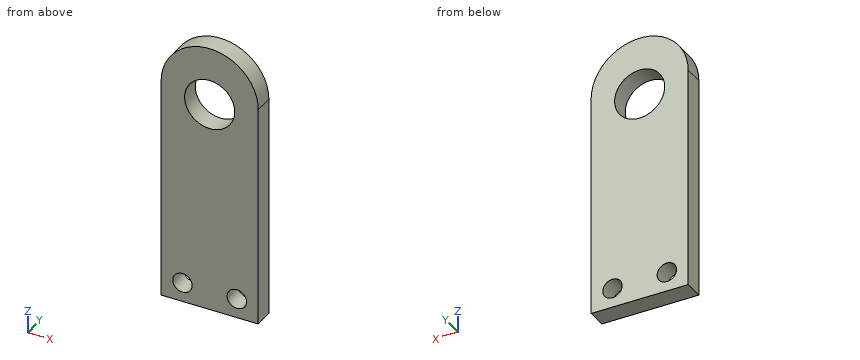
Autodesk Inventor part; units mm, degrees
ref_plane "YZ Plane" through (0, 0, 0) normal (1, 0, 0) x (0, 1, 0)
ref_plane "XZ Plane" through (0, 0, 0) normal (0, 1, 0) x (-1, 0, 0)
ref_plane "XY Plane" through (0, 0, 0) normal (0, 0, 1) x (1, 0, 0)
sketch "Sketch1" plane through (0, 0, 0) normal (0, 1, 0) x (-1, 0, 0)
  line L0 (22.1143, 19.9744) -> (22.1143, -53.0506)
  line L1 (22.1143, -53.0506) -> (-9.6357, -53.0506)
  line L2 (-9.6357, -53.0506) -> (-9.6357, 19.9744)
  arc A0 (22.1143, 19.9744) -> (-9.6357, 19.9744) centre (6.2393, 19.9744) ccw
  circle A1 centre (15.1293, -46.7006) radius 3.175
  circle A2 centre (-2.6507, -46.7006) radius 3.175
  circle A3 centre (6.2393, 16.7994) radius 8.1915
  point P0 (0, 0)
  point P1 (6.2393, 35.8494)
  dimension "d0" = 31.75
  dimension "d1" = 88.9
  dimension "d3" = 6.35
  dimension "d4" = 6.35
  dimension "d5" = 17.78
  dimension "d6" = 6.35
  dimension "d7" = 6.35
  dimension "d10" = 6.985
  dimension "d11" = 6.985
  dimension "d12" = 16.383
  dimension "d14" = 3.175
  dimension "d15" = 15.875
  dimension "d16" = 15.875
extrude "Extrusion2" add sketch "Sketch1" along normal blind 6.35
equation "\"d7\" = d6"
equation "\"d10\" = d11"
equation "\"d15\" = d16"
properties part number "self aligning bearing holder"
Part model, mm, in its own coordinate system. Coordinates: 2 decimals unless noted, no trailing zeros. Loops run counter-clockwise (first coordinate to the right, second up) from the corner with the lowest first, then second, coordinate; pieces in that order, holes last. Notation, with made-up numbers: (-15.5, 29.25) - (13.5, 29.25) arc R20 cw to (13.5, 39.25) - close; hole circle Ø9 at (82, 2.5). An arc over 180 degrees is marked (long way). Write each question's results on one line, items separated by ' | '. Start each with the question number.
Q1. Slice it at C-C on y = 1.25. Give the number of separate pieces and of enclosed holes in the cut face, and give its area (3 significant figures).
Q2. Probe line 1 along Z through (x, y) = (1, 2.75); line 2 along X through (y, z) = (2.75, 15); line 3 along X through (y, z) = (6.25, 13.5). List the from-to ranges inside material, lowest first.
Q3. Slice it at A-A on x = -2. Give the cut face in (y, z).
Q4. Slice it at D-D on z = 26.5. Give the cut face in (x, y).
Q5. Slice it at B-B on z = 12.5. Give the cut face in (x, y), and give its area (3 significant figures).
Answer:
1) separate pieces: 1 | enclosed holes: 3 | area: 2,440 mm2
2) line 1: z = -53.05 to -49.41, -43.99 to 12.97, 20.63 to 34.1 | line 2: x = -22.11 to -14.23, 1.75 to 9.64 | line 3: x = -22.11 to -13.74, 1.26 to 9.64
3) outline: (0, -53.05) - (6.35, -53.05) - (6.35, 9.79) - (0, 9.79) - close; (0, 23.81) - (6.35, 23.81) - (6.35, 35.27) - (0, 35.27) - close
4) outline: (-20.71, 0) - (8.23, 0) - (8.23, 6.35) - (-20.71, 6.35) - close
5) outline: (-22.11, 0) - (-13.21, 0) - (-13.21, 6.35) - (-22.11, 6.35) - close; (0.73, 0) - (9.64, 0) - (9.64, 6.35) - (0.73, 6.35) - close | area: 113 mm2
